Design review of the part built by this model. Coordinates are the model's own, in mm. Face numbers are marked on the shaded views. Give positions to 0.01 mm unless a question says otherwise; leave off trailing zeros. Write each loop counter-clockwise with the first axis right and the second up, starting at its lowest first coordinate (ties: lowest second). Pieces come first, ordered by that corner, then holes. Notation, with made-up numbers: (67, 85.25) -> (116, 85.25) arc R14 ccw to (116, 108.25) -> close; hole circle Ø2 at (36.25, 53). An arc over 180 degrees is marked (long way). Write each question's results on one line, items separated by ' | '. Start each with the question number.
(1) Take a section at C-C (x = 10.5). State the section outline as (y, z) points, plus the area to 3 significant figures.
(2) Mouldability with a two-part tool opening along Y and no side actions: class the marked faces 1, 2 and 3 as released by +Y, released by -Y, zero draft, split by the parting line, or undercut.
(3) Take a section at A-A (z = 0). State the section outline as (x, y) points, plus the area to 3 significant figures.
(4) Clearance check with a flat-ended pin moving along its axis: pin 1 (8 mm diameter, centred on y = 16.5, z = 6.5, fed in from +X). State where the tip first meets the part, or that it passes through.
(5) To check wall thickness, follow probe 1 along Y at (x, z) = (58, 0); probe 2 along Z at (x, y) = (65, -1); probe 3 along Y at (x, z) = (55.5, -21.5). State the ranges of each line that lie inside material, in increasing order.
(6) Take a section at D-D (z = 50.5). State the section outline as (x, y) points, plus the area to 3 significant figures.
(7) Take a section at B-B (y = 0). State the section outline as (x, z) points, plus the area to 3 significant figures.
from build123d import *

# Parameters (mm, degrees)
CROQUIS2_R              = 25.4
SALIENTE_EXTRUIR1_DEPTH = 127


with BuildPart() as part:
    # Croquis2 → Saliente-Extruir1 (new body)
    with BuildSketch(Plane.YZ):
        with BuildLine():
            Line((-101.6, 63.5), (101.6, 63.5))
            ThreePointArc((101.6, 63.5), (119.560512242, 56.060512242), (127, 38.1))
            Line((127, 38.1), (127, -38.1))
            ThreePointArc((127, -38.1), (119.560512242, -56.060512242), (101.6, -63.5))
            Line((101.6, -63.5), (-101.6, -63.5))
            ThreePointArc((-101.6, -63.5), (-119.560512242, -56.060512242), (-127, -38.1))
            Line((-127, -38.1), (-127, 38.1))
            ThreePointArc((-127, 38.1), (-119.560512242, 56.060512242), (-101.6, 63.5))
        make_face()
        with Locations(Location((0, 0, 0), (0, 0, 270))):
            Circle(CROQUIS2_R, mode=Mode.SUBTRACT)
    extrude(amount=SALIENTE_EXTRUIR1_DEPTH)


solid = part.part
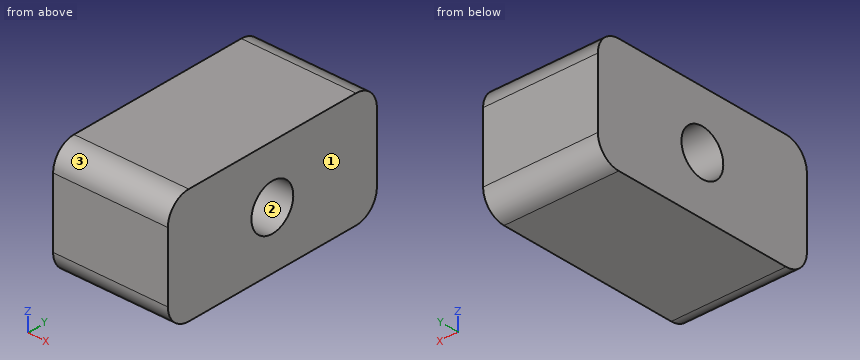
Report:
1) outline: (-127, -38.1) arc R25.4 ccw to (-101.6, -63.5) -> (101.6, -63.5) arc R25.4 ccw to (127, -38.1) -> (127, 38.1) arc R25.4 ccw to (101.6, 63.5) -> (-101.6, 63.5) arc R25.4 ccw to (-127, 38.1) -> close; hole circle Ø50.8 at (0, 0) | area: 29,700 mm2
2) face 1: zero draft | face 2: undercut | face 3: released by -Y
3) outline: (0, -127) -> (127, -127) -> (127, -25.4) -> (0, -25.4) -> close; (0, 25.4) -> (127, 25.4) -> (127, 127) -> (0, 127) -> close | area: 25,800 mm2
4) pin 1: through
5) probe 1: -127 to -25.4, 25.4 to 127 | probe 2: -63.5 to -25.38, 25.38 to 63.5 | probe 3: -127 to -13.52, 13.52 to 127
6) outline: (0, -123.77) -> (127, -123.77) -> (127, 123.77) -> (0, 123.77) -> close | area: 31,400 mm2
7) outline: (0, -63.5) -> (127, -63.5) -> (127, -25.4) -> (0, -25.4) -> close; (0, 25.4) -> (127, 25.4) -> (127, 63.5) -> (0, 63.5) -> close | area: 9,680 mm2
